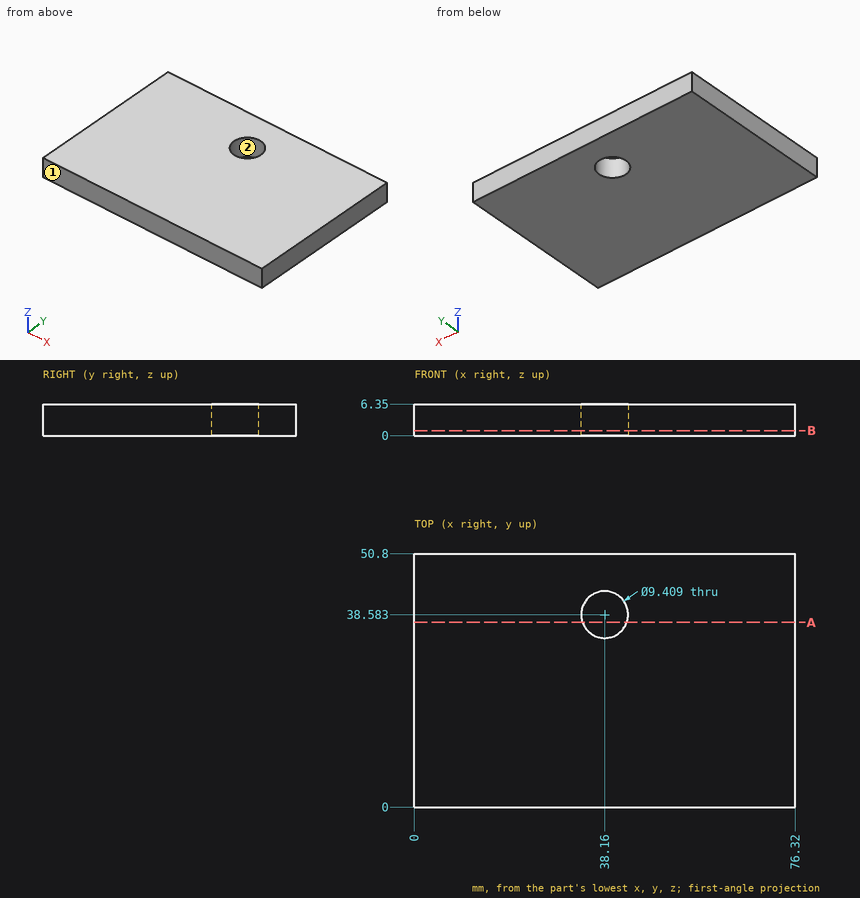
For this review, use the dimensioned drawing (mm, ordinates from the lowest corner) and the shaded views. Give positions to 0.01 mm unless a question says otherwise; leave off trailing zeros. Order: outer loops, then holes, each group sorted by start corner. A loop starts at its lowest first (then second) coordinate and runs counter-clockwise, first axis right, second up.
1. To check wall thickness, follow L1, parallel to X at y = 40, z = 2; L2, parallel to X at y = 35.5, z = 2 (1 decimal); L3, parallel to Y at x = 40, z = 2. State the ranges of each line that lie inside material, in increasing order.
Solution:
L1: x = 0 to 33.67, 42.65 to 76.32
L2: x = 0 to 34.6, 41.7 to 76.3
L3: y = 0 to 34.25, 42.91 to 50.8
2. Add section B-B, the plane z = 1. State the section outline as (x, y) points (1 decimal), then the cut area to 3 significant figures.
Solution:
outline: (0, 0) - (76.3, 0) - (76.3, 50.8) - (0, 50.8) - close; hole circle Ø9.4 at (38.2, 38.6)
area: 3,810 mm2
3. Mouldability with a two-part tool opening along X and no side actions: class the marked faces 1 and 2 as +X half, -X half, draft (parallel to the pull), parting line (faces both ways), or undercut.
Solution:
face 1: draft
face 2: undercut
4. Add section A-A, the plane y = 37. State the section outline as (x, z) points, then the cut area to 3 significant figures.
Solution:
outline: (0, 0) - (33.73, 0) - (33.73, 6.35) - (0, 6.35) - close; (42.59, 0) - (76.32, 0) - (76.32, 6.35) - (42.59, 6.35) - close
area: 428 mm2
